Can you work these out from the model? Positions are in its coordinate system, mm. A direction names the side the tool comes from. Coordinates: 2 decimals unless noted, no trailing zeros. Order: outer loops, then holes, each group sorted by start corner. A loop starts at its lowest first (then second) coordinate and runs counter-clockwise, first axis right, second up. Notation, with made-up numbers: M 35.25,7.5 L 89.25,7.5 A32 cw 89.25,34.5 Z; hole C -7.75,30 d1. An arc over 180 degrees is marked long. Answer as CSV lines item,"result". Start each with the question number.
1. If we section it at D-D (x = 16.5): List the corners of the cut face in (y, z) for me.
2. If we section it at A-A (x = 5): List the corners of the cut face in (y, z) for me, plus the area to 3 significant figures.
3. Will these pins go through, and if not, where does the flat tip stop? pin 1 (8 mm diameter, centred on x = 4, y = 21.5, fed in from -Z); pin 2 (3 mm diameter, centred on y = 26.5, z = -15, fed in from -X).
4. If we section it at B-B (y = 18.75): List the corners of the cut face in (x, z) for me, plus the area to 3 significant figures.
5. On a 3-axis mill with a long thin cutter (end or side, diameter ignored), from which of +Z, -Z, +X, -X, +Y, -Y can I reach the whole of each face in a straight line? I mean faces 4 (the face through (20, 15, -18)), 5 (the face through (5, 15, 0)), 6 (the face through (15, 25.16, -26)). Say none if no direction works.
6. I need wall thicknesses on line 1 along Y through (x, z) = (5, 0.5); line 2 along Z through (x, y) = (17.5, 12.25); line 3 along Y through (x, z) = (12.5, -28.5). Which ranges of each line are inside material? Lowest first, please. Write a range as from..to.
7. If we section it at C-C (z = -10.5): List the corners of the cut face in (x, y) for me, plus the area to 3 significant figures.
8. If we mould it in two halves opening along X, with no side actions, what happens to faces 1 (the face through (0, 15, 1)), 2 (the face through (15, 30, -13)), 3 (the face through (4.697, 23.633, 1.252))? For each: released by +X, released by -X, zero draft, split by the parting line, or undercut.
```python
from build123d import *

# Parameters (mm, degrees)
SKETCH2_W           = 30
SKETCH2_H           = 30
SKETCH2_R           = 1.4
BOSS_EXTRUDE1_DEPTH = 2.54
SKETCH3_W           = 10
SKETCH3_H           = 30
BOSS_EXTRUDE2_DEPTH = 35.56
SKETCH4_W           = 8.763
SKETCH4_H           = 20.32
CUT_EXTRUDE1_DEPTH  = 35.56


with BuildPart() as part:
    # Sketch2 → Boss-Extrude1 (new body)
    with BuildSketch(Plane.XY):
        with Locations((15, 15)):
            Rectangle(SKETCH2_W, SKETCH2_H)
        with Locations((5, 5)):
            Circle(SKETCH2_R, mode=Mode.SUBTRACT)
        with Locations((25, 5)):
            Circle(SKETCH2_R, mode=Mode.SUBTRACT)
        with Locations((5, 25)):
            Circle(SKETCH2_R, mode=Mode.SUBTRACT)
        with Locations((25, 25)):
            Circle(SKETCH2_R, mode=Mode.SUBTRACT)
    extrude(amount=BOSS_EXTRUDE1_DEPTH)

    # Sketch3 → Boss-Extrude2 (add)
    with BuildSketch(Plane(origin=(0, 0, 0), x_dir=(-1, 0, 0), z_dir=(0, 0, -1))):
        with Locations((-15, 15)):
            Rectangle(SKETCH3_W, SKETCH3_H)
    extrude(amount=BOSS_EXTRUDE2_DEPTH)

    # Sketch4 → Cut-Extrude1 (cut)
    with BuildSketch(Plane.ZY.offset(-10)):
        with Locations((-25.8445, 15)):
            Rectangle(SKETCH4_W, SKETCH4_H)
        with Locations((-12.0015, 15)):
            Rectangle(SKETCH4_W, SKETCH4_H)
    extrude(amount=-CUT_EXTRUDE1_DEPTH, mode=Mode.SUBTRACT)


solid = part.part
```
Solved:
1,outline,"M 0,-35.56 L 30,-35.56 L 30,2.54 L 0,2.54 Z; hole M 4.84,-30.23 L 25.16,-30.23 L 25.16,-21.46 L 4.84,-21.46 Z; hole M 4.84,-16.38 L 25.16,-16.38 L 25.16,-7.62 L 4.84,-7.62 Z"
2,outline,"M 0,0 L 3.6,0 L 3.6,2.54 L 0,2.54 Z; M 6.4,0 L 23.6,0 L 23.6,2.54 L 6.4,2.54 Z; M 26.4,0 L 30,0 L 30,2.54 L 26.4,2.54 Z"
2,area,"62.0 mm²"
3,pin 1,"z = 0"
3,pin 2,"x = 10"
4,outline,"M 0,0 L 10,0 L 10,-7.62 L 20,-7.62 L 20,0 L 30,0 L 30,2.54 L 0,2.54 Z; M 10,-35.56 L 20,-35.56 L 20,-30.23 L 10,-30.23 Z; M 10,-21.46 L 20,-21.46 L 20,-16.38 L 10,-16.38 Z"
4,area,"257 mm²"
5,face 4,"-Z, +X, +Y, -Y"
5,face 5,"-Z, -X, +Y, -Y"
5,face 6,"+X, -X"
6,line 1,"0..3.6, 6.4..23.6, 26.4..30"
6,line 2,"-35.56..-30.23, -21.46..-16.38, -7.62..2.54"
6,line 3,"0..4.84, 25.16..30"
7,outline,"M 10,0 L 20,0 L 20,4.84 L 10,4.84 Z; M 10,25.16 L 20,25.16 L 20,30 L 10,30 Z"
7,area,"96.8 mm²"
8,face 1,"released by -X"
8,face 2,"zero draft"
8,face 3,"undercut"
